Verification items for the finished model (mm, model axes). A direction names the side the tool comes from. Coordinates: 2 decimals unless noted, no trailing zeros. Write each loop counter-clockwise with the first axis right and the second up, starting at its lowest first coordinate (ties: lowest second). Pieces come first, ordered by that corner, then holes. Notation, with made-up numbers: (-35, 81) -> (17, 81) arc R16 ccw to (17, 97) -> close; hole circle Ø7 at (26, 53.5). An arc over 180 degrees is marked (long way). Write item = value, one per line. Start each with the question number.
(1) Section check B-B (y = 1.8). Record the cut outline in (x, z).
(2) Gauge pin test, flat ends, axial feed: pin 1 Ø2 at (y, z) = (2.5, 62.5) entering from +X; pin 2 Ø2 at (y, z) = (1, 124) entering from -X; pin 3 Ø1 at (y, z) = (3, 155) entering from -X. Record the tip position at first contact, or that the pin passes through.
(3) Section check D-D (x = 91). Record the cut outline in (y, z), plus the area to 3 significant figures.
(4) Set-up check for faces 4 (the face through (-19.483, 1.972, 142.39)), 5 (the face through (-36.499, 1.972, 160.728)): record each of +Z, -Z, +X, -X, +Y, -Y from which the full face is reachable in a straight line by a thin tool's end or side.
(5) Mould release check, pull along X, two halves, no side actions. Record for faces 1 (the face through (244.8, 1.97, 8.01)), 2 (the face through (-37.354, 1.972, -6.309)), 3 (the face through (266.31, 1.97, 159.87)): released by +X, released by -X, zero draft, split by the parting line, or undercut.
(6) Material ranges on probe 1 along Z at (x, y) = (178, 2.45); probe 2 along Z at (x, y) = (202, 1.8); probe 3 along Z at (x, y) = (92.5, 3.45), recorded low to high. Write a range as [from, to].
(7) Section check A-A (z = 113). Record the cut outline in (x, y).
(8) Section check C-C (x = 222.5). Record the cut outline in (y, z).
```python
from build123d import *

# Parameters (mm, degrees)
BOSS_EXTRUDE1_DEPTH = 4


with BuildPart() as part:
    # Sketch1 → Boss-Extrude1 (new body)
    with BuildSketch(Plane(origin=(0, 0, 0), x_dir=(1, 0, 0), z_dir=(0, 1, 0))):
        with BuildLine():
            Line((281.992313692, -105.781584964), (281.992313692, -121.411584964))
            ThreePointArc((281.992313692, -121.411584964), (265.883186657, -160.302457929), (226.992313692, -176.411584964))
            Line((226.992313692, -176.411584964), (1.962313692, -176.411584964))
            ThreePointArc((1.962313692, -176.411584964), (-36.928559274, -160.302457929), (-53.037686308, -121.411584964))
            Line((-53.037686308, -121.411584964), (-53.037686308, -32.151584964))
            ThreePointArc((-53.037686308, -32.151584964), (-36.928559274, 6.739288001), (1.962313692, 22.848415036))
            Line((1.962313692, 22.848415036), (226.992313692, 22.848415036))
            ThreePointArc((226.992313692, 22.848415036), (265.883186657, 6.739288001), (281.992313692, -32.151584964))
            Line((281.992313692, -32.151584964), (281.992313692, -47.781584964))
            Line((281.992313692, -47.781584964), (194.992313692, -47.781584964))
            Line((194.992313692, -47.781584964), (194.992313692, -105.781584964))
            Line((194.992313692, -105.781584964), (281.992313692, -105.781584964))
        make_face()
        with BuildLine():
            Line((1.962313692, -151.411584964), (226.992313692, -151.411584964))
            ThreePointArc((226.992313692, -151.411584964), (244.583504669, -145.712819501), (255.491490873, -130.781584964))
            Line((255.491490873, -130.781584964), (169.992313692, -130.781584964))
            Line((169.992313692, -130.781584964), (169.992313692, -22.781584964))
            Line((169.992313692, -22.781584964), (255.491490873, -22.781584964))
            ThreePointArc((255.491490873, -22.781584964), (244.583504669, -7.850350427), (226.992313692, -2.151584964))
            Line((226.992313692, -2.151584964), (1.962313692, -2.151584964))
            ThreePointArc((1.962313692, -2.151584964), (-19.250889744, -10.938381528), (-28.037686308, -32.151584964))
            Line((-28.037686308, -32.151584964), (-28.037686308, -121.411584964))
            ThreePointArc((-28.037686308, -121.411584964), (-19.250889744, -142.6247884), (1.962313692, -151.411584964))
        make_face(mode=Mode.SUBTRACT)
    extrude(amount=BOSS_EXTRUDE1_DEPTH)


solid = part.part
```
Response:
q1.outline = (-53.04, 32.15) arc R55 ccw to (1.96, -22.85) -> (226.99, -22.85) arc R55 ccw to (281.99, 32.15) -> (281.99, 47.78) -> (194.99, 47.78) -> (194.99, 105.78) -> (281.99, 105.78) -> (281.99, 121.41) arc R55 ccw to (226.99, 176.41) -> (1.96, 176.41) arc R55 ccw to (-53.04, 121.41) -> close; hole (-28.04, 32.15) arc R30 ccw to (1.96, 2.15) -> (226.99, 2.15) arc R30 ccw to (255.49, 22.78) -> (169.99, 22.78) -> (169.99, 130.78) -> (255.49, 130.78) arc R30 ccw to (226.99, 151.41) -> (1.96, 151.41) arc R30 ccw to (-28.04, 121.41) -> close
q2.pin_1 = 194.99
q2.pin_2 = -53.01
q2.pin_3 = -41.97
q3.outline = (0, -22.85) -> (4, -22.85) -> (4, 2.15) -> (0, 2.15) -> close; (0, 151.41) -> (4, 151.41) -> (4, 176.41) -> (0, 176.41) -> close
q3.area = 200 mm2
q4.face_4 = +Y, -Y
q4.face_5 = +Z, -X, +Y, -Y
q5.face_1 = undercut
q5.face_2 = released by -X
q5.face_3 = released by +X
q6.probe_1 = [-22.85, 2.15], [22.78, 130.78], [151.41, 176.41]
q6.probe_2 = [-22.85, 2.15], [22.78, 47.78], [105.78, 130.78], [151.41, 176.41]
q6.probe_3 = [-22.85, 2.15], [151.41, 176.41]
q7.outline = (-53.04, 0) -> (-28.04, 0) -> (-28.04, 4) -> (-53.04, 4) -> close; (169.99, 0) -> (281.99, 0) -> (281.99, 4) -> (169.99, 4) -> close
q8.outline = (0, -22.85) -> (4, -22.85) -> (4, 2.15) -> (0, 2.15) -> close; (0, 22.78) -> (4, 22.78) -> (4, 47.78) -> (0, 47.78) -> close; (0, 105.78) -> (4, 105.78) -> (4, 130.78) -> (0, 130.78) -> close; (0, 151.41) -> (4, 151.41) -> (4, 176.41) -> (0, 176.41) -> close
